```python
from build123d import *

# Parameters (mm, degrees)
MODEL_R            = 2.1
BOSS_EXTRU_1_DEPTH = 8
CHANFREIN1_SIZE    = 1


with BuildPart() as part:
    # Model → Boss.-Extru.1 (new body)
    with BuildSketch(Plane.XY):
        with BuildLine():
            Line((-24.192398664, -96.552630985), (-24.192398664, -106.552630985))
            ThreePointArc((-24.192398664, -106.552630985), (-21.263466476, -113.623698797), (-14.192398664, -116.552630985))
            Line((-14.192398664, -116.552630985), (1.807601336, -116.552630985))
            ThreePointArc((1.807601336, -116.552630985), (4.636028461, -117.72420386), (5.807601336, -120.552630985))
            Line((5.807601336, -120.552630985), (5.807601336, -137.552630985))
            ThreePointArc((5.807601336, -137.552630985), (6.979174211, -140.38105811), (9.807601336, -141.552630985))
            Line((9.807601336, -141.552630985), (72.853374331, -141.552630985))
            ThreePointArc((72.853374331, -141.552630985), (77.007626671, -139.831883325), (78.728374331, -135.677630985))
            Line((78.728374331, -135.677630985), (78.728374331, -67.427630985))
            ThreePointArc((78.728374331, -67.427630985), (77.007626671, -63.273378646), (72.853374331, -61.552630985))
            Line((72.853374331, -61.552630985), (9.807601336, -61.552630985))
            ThreePointArc((9.807601336, -61.552630985), (6.979174211, -62.72420386), (5.807601336, -65.552630985))
            Line((5.807601336, -65.552630985), (5.807601336, -82.552630985))
            ThreePointArc((5.807601336, -82.552630985), (4.636028461, -85.38105811), (1.807601336, -86.552630985))
            Line((1.807601336, -86.552630985), (-14.192398664, -86.552630985))
            ThreePointArc((-14.192398664, -86.552630985), (-21.263466476, -89.481563173), (-24.192398664, -96.552630985))
        make_face()
        with Locations((22.853374331, -68.052630985)):
            Circle(MODEL_R, mode=Mode.SUBTRACT)
        with Locations((72.853374331, -68.052630985)):
            Circle(MODEL_R, mode=Mode.SUBTRACT)
        with Locations((29.048492507, -93.052630985)):
            Circle(MODEL_R, mode=Mode.SUBTRACT)
        with Locations((29.048492507, -110.052630985)):
            Circle(MODEL_R, mode=Mode.SUBTRACT)
        with Locations((49.048492507, -93.052630985)):
            Circle(MODEL_R, mode=Mode.SUBTRACT)
        with Locations((49.048492507, -110.052630985)):
            Circle(MODEL_R, mode=Mode.SUBTRACT)
        with Locations((69.048492507, -93.052630985)):
            Circle(MODEL_R, mode=Mode.SUBTRACT)
        with Locations((69.048492507, -110.052630985)):
            Circle(MODEL_R, mode=Mode.SUBTRACT)
        with Locations((22.853374331, -135.052630985)):
            Circle(MODEL_R, mode=Mode.SUBTRACT)
        with Locations((72.853374331, -135.052630985)):
            Circle(MODEL_R, mode=Mode.SUBTRACT)
        with BuildLine():
            Line((15.807601336, -137.214613672), (15.807601336, -119.214613672))
            ThreePointArc((15.807601336, -119.214613672), (14.807601336, -118.214613672), (13.807601336, -119.214613672))
            Line((13.807601336, -119.214613672), (13.807601336, -137.214613672))
            ThreePointArc((13.807601336, -137.214613672), (14.807601336, -138.214613672), (15.807601336, -137.214613672))
        make_face(mode=Mode.SUBTRACT)
        with BuildLine():
            Line((15.807601336, -65.890648299), (15.807601336, -83.890648299))
            ThreePointArc((15.807601336, -83.890648299), (14.807601336, -84.890648299), (13.807601336, -83.890648299))
            Line((13.807601336, -83.890648299), (13.807601336, -65.890648299))
            ThreePointArc((13.807601336, -65.890648299), (14.807601336, -64.890648299), (15.807601336, -65.890648299))
        make_face(mode=Mode.SUBTRACT)
        with BuildLine():
            Line((-8.692398664, -97.552630985), (1.307601336, -97.552630985))
            ThreePointArc((1.307601336, -97.552630985), (5.307601336, -101.552630985), (1.307601336, -105.552630985))
            Line((1.307601336, -105.552630985), (-8.692398664, -105.552630985))
            ThreePointArc((-8.692398664, -105.552630985), (-12.692398664, -101.552630985), (-8.692398664, -97.552630985))
        make_face(mode=Mode.SUBTRACT)
    extrude(amount=BOSS_EXTRU_1_DEPTH)

    # Chanfrein1
    chanfrein1_edges = [part.edges().sort_by_distance(p)[0] for p in [
        (14.807601336, -118.214613672, 0),
        (13.807601336, -128.214613672, 0),
        (14.807601336, -138.214613672, 0),
        (15.807601336, -128.214613672, 0),
        (14.807601336, -118.214613672, 8),
        (13.807601336, -128.214613672, 8),
        (14.807601336, -138.214613672, 8),
        (15.807601336, -128.214613672, 8),
        (20.753374331, -68.052630985, 8),
        (70.753374331, -68.052630985, 8),
        (26.948492507, -93.052630985, 8),
        (26.948492507, -110.052630985, 8),
        (46.948492507, -93.052630985, 8),
        (46.948492507, -110.052630985, 8),
        (66.948492507, -93.052630985, 8),
        (66.948492507, -110.052630985, 8),
        (20.753374331, -135.052630985, 8),
        (70.753374331, -135.052630985, 8),
        (14.807601336, -64.890648299, 0),
        (13.807601336, -74.890648299, 0),
        (14.807601336, -84.890648299, 0),
        (15.807601336, -74.890648299, 0),
        (14.807601336, -64.890648299, 8),
        (13.807601336, -74.890648299, 8),
        (14.807601336, -84.890648299, 8),
        (15.807601336, -74.890648299, 8),
    ]]
    chamfer(chanfrein1_edges, length=CHANFREIN1_SIZE)


solid = part.part
```
Geometry check sheet. Reference: the model listing, model coordinates, mm. A direction names the side the tool comes from. Coordinates: 2 decimals unless noted, no trailing zeros. Loops run counter-clockwise (first coordinate to the right, second up) from the corner with the lowest first, then second, coordinate; pieces in that order, holes last.
Item 1: Sectioned sample at B-B, the plane z = 3.75. Count the separate pieces of the cut face and the enclosed holes in it, then the cut area to 3 significant figures.
Item 2: Sectioned sample at A-A, the plane y = -127. Record the boundary of the cut face in (x, z), then the cut area to 3 significant figures.
Item 3: Sectioned sample at D-D, the plane x = -18. Record the boundary of the cut face in (y, z).
Item 4: Go/stop test with flat-tipped pins: pin 1 Ø2.5 at (x, z) = (-10, 4) entering from -Y; pin 2 Ø5 at (x, y) = (49.05, -110.05) entering from +Z; pin 3 Ø3 at (y, z) = (-74, 5.5) entering from -X. Record where each tip stops, or that it passes through.
Item 5: Thickness scan on line 1 (Y direction, x = -1, z = 1.75); line 2 (Y direction, x = 23.5, z = 3.25); line 3 (Y direction, x = -9, z = 2.5). Record the ranges inside material, lowest first.
Item 6: Release check for a two-part mould opening along X. For faces 1 (the face through (5.808, -74, 4)), 2 (the face through (76.96, -139.88, 3.94)), 3 (the face through (14.779, -138.499, 7.285)) record: released by +X, released by -X, zero draft, split by the parting line, or undercut.
Item 7: Access from +Z, -Z, +X, -X, +Y, -Y to the whole of each face (thin tool, end or side, straight path). Record for faces 4 (the face through (15.808, -128, 4)), 5 (the face through (14.836, -117.93, 7.285)), 6 (the face through (-6, -116.553, 4)), 7 (the face through (38, -101, 0)).
Check result:
1. separate pieces: 1
1. enclosed holes: 13
1. area: 6,330 mm2
2. outline: (5.81, 0) - (12.81, 0) - (13.81, 1) - (13.81, 7) - (12.81, 8) - (5.81, 8) - close; (15.81, 1) - (16.81, 0) - (78.73, 0) - (78.73, 8) - (16.81, 8) - (15.81, 7) - close
2. area: 565 mm2
3. outline: (-115.8, 0) - (-87.31, 0) - (-87.31, 8) - (-115.8, 8) - close
4. pin 1: stops at y = -116.55
4. pin 2: stops at z = 7.4
4. pin 3: stops at x = 5.81
5. line 1: y = -116.55 to -105.55, -97.55 to -86.55
5. line 2: y = -141.55 to -137.05, -133.05 to -70.05, -66.05 to -61.55
5. line 3: y = -116.55 to -105.54, -97.56 to -86.55
6. face 1: released by -X
6. face 2: released by +X
6. face 3: undercut
7. face 4: +Z, -Z
7. face 5: +Z
7. face 6: +Z, -Z, -X, -Y
7. face 7: -Z, +X, -X, +Y, -Y
